Can you work these out from the model? Positions are in its coordinate system, mm. A direction names the side the tool comes from. Round coordinates to 2 decimals unless told otherwise and drop trailing zeros. Write each loop counter-clockwise with the first axis right and the second up, starting at its lowest first coordinate (ties: lowest second). Pieces come first, ordered by that corner, then holes. Notation, with made-up numbers: M 52,33 L 100,33 A20 ccw 100,72 Z; hole C -39.5,67 d5. An arc over 180 degrees is marked long. Answer in a Markdown table with one row per item. Add a question column.
(1) I'm going to push a flat-ended pin straight in: pin 1 (23 mm diameter, centred on x = 4, y = -7, fed in from +Z). Where does the tip first touch, or does it pass through?
(2) If I drill on probe 1 along Z at (x, y) = (-9, -10.5); probe 2 along Y at (x, z) = (14.5, -28.5); probe 3 along X at (y, z) = (0, -47), over which ranges is the centre line in solid material (lowest first)?
(3) Suppose I cut it at A-A, the plane z = -31. Write out the boundary of the cut face in (x, y).
(4) If we mould it in two halves opening along Y, with no side actions, what happens to faces 5 (the face through (-18, 24.25, -52)), 6 (the face through (-18, -24.25, -52)), 7 (the face through (-1, 0, -135)), 8 (the face through (-21.245, 0.467, -115.172))? For each: released by +Y, released by -Y, zero draft, split by the parting line, or undercut.
(5) Suppose I cut it at B-B, the plane x = 7. Count the separate pieces of the cut face and the enclosed holes in it, then the cut area to 3 significant figures.
(6) For faces 1 (the face through (22, 0, -32.5)), 2 (the face through (1, 0, -130)), 3 (the face through (-21.23, 0.93, -20.04)), 4 (the face through (-26.25, 0, -67)), which set-ups out of +Z, -Z, +X, -X, +Y, -Y let a thin tool reach every point of the face, with its end or its side?
(7) Suppose I cut it at C-C, the plane z = -80. Write out the boundary of the cut face in (x, y).
from build123d import *

# Parameters (mm, degrees)
F1_DEPTH      = 135
F2_R          = 21.25
F3_DEPTH      = 130
F4_W          = 24.25
F4_H          = 97.5
F5_DEPTH      = 50.1
F5_DEPTH_BACK = 25
F6_R          = 1.49999
F7_T3_DEPTH   = 141.00001
F7_T6_DEPTH   = 56
F7_T9_DEPTH   = 141.00001
F8_T1_DEPTH   = 28.5
F8_T4_ANGLE   = 180


# Not quite as in the source:
# - a fillet or chamfer that OpenCascade refuses, or shapes differently, is made with other operations: its cross-section is extruded or revolved along the edge and cut away or added
# - a fillet or chamfer is up to 0.001 mm smaller than in the source, because OpenCascade refuses the exact size


with BuildPart() as f1:
    # F0 (on Top) → F1 (new body)
    with BuildSketch(Plane.XY):
        with BuildLine():
            ThreePointArc((0, -24.25), (17.1473394438, -17.1473394438), (24.25, 0))
            ThreePointArc((24.25, 0), (17.1473394438, 17.1473394438), (0, 24.25))
            ThreePointArc((0, 24.25), (-24.25, 0), (0, -24.25))
        make_face()
        with BuildLine():
            ThreePointArc((0, -24.25), (-24.25, 0), (0, 24.25))
            Line((0, 24.25), (-26.25, 24.25))
            Line((-26.25, 24.25), (-26.25, -24.25))
            Line((-26.25, -24.25), (0, -24.25))
        make_face()
    extrude(amount=-F1_DEPTH)

    # F2 (on face) → F3 (cut)
    with BuildSketch(Plane.XY):
        Circle(F2_R)
    extrude(amount=-F3_DEPTH, mode=Mode.SUBTRACT)

    # F4 (on face) → F5 (cut, two sides)
    with BuildSketch(Plane.XZ.offset(24.25)) as f5_sk:
        with Locations((12.125, -81.25)):
            Rectangle(F4_W, F4_H)
        with BuildLine():
            Line((0, -130), (0, -32.5))
            ThreePointArc((0, -32.5), (-22.2460263089, -81.25), (0, -130))
        make_face()
    extrude(amount=-F5_DEPTH, mode=Mode.SUBTRACT)
    extrude(f5_sk.sketch, amount=F5_DEPTH_BACK, mode=Mode.SUBTRACT)

    # F6 (radius 1.5 in the source; OpenCascade refuses exactly that, so slightly less here)
    f6_edges = [f1.edges().sort_by_distance(p)[0] for p in [
        (24.25, 0, 0),
        (-13.125, -24.25, 0),
        (-13.125, 24.25, 0),
        (-26.25, 0, 0),
        (-21.25, 0, 0),
    ]]
    fillet(f6_edges, radius=F6_R)

    # F7: fillet of radius 1.5 on 4 edges, made by hand


with BuildPart() as f7_tool1:
    # F7_s2 → F7_t3 (new body)
    with BuildSketch(Plane.XY.offset(2.25001)):
        with BuildLine():
            ThreePointArc((-24.75, 24.25), (-25.8106601718, 23.8106601718), (-26.25, 22.75))
            Line((-26.25, 22.75), (-26.25, 24.25))
            Line((-26.25, 24.25), (-24.75, 24.25))
        make_face()
    extrude(amount=-F7_T3_DEPTH)


with BuildPart() as f7_tool4:
    # F7_s5 → F7_t6 (new body)
    with BuildSketch(Plane.XZ.offset(-28)):
        with BuildLine():
            ThreePointArc((-26.25, -133.5), (-25.8106601718, -134.5606601718), (-24.75, -135))
            Line((-24.75, -135), (-26.25, -135))
            Line((-26.25, -135), (-26.25, -133.5))
        make_face()
    extrude(amount=F7_T6_DEPTH)


with BuildPart() as f7_tool7:
    # F7_s8 → F7_t9 (new body)
    with BuildSketch(Plane.XY.offset(2.25001)):
        with BuildLine():
            ThreePointArc((-24.75, -24.25), (-25.8106601718, -23.8106601718), (-26.25, -22.75))
            Line((-26.25, -22.75), (-26.25, -24.25))
            Line((-26.25, -24.25), (-24.75, -24.25))
        make_face()
    extrude(amount=-F7_T9_DEPTH)


with BuildPart() as f1_1:
    add(f1.part)

    # F7_t10: cut F7_tool1, F7_tool4, F7_tool7
    add([f7_tool1.part, f7_tool4.part, f7_tool7.part], mode=Mode.SUBTRACT)

    # F8: fillet of radius 1.5 on 4 edges, made by hand

    # F8_s2 → F8_t1 (cut)
    with BuildSketch(Plane.YZ.offset(-28.5)):
        with BuildLine():
            ThreePointArc((-24.25, -133.5), (-23.8106601718, -134.5606601718), (-22.75, -135))
            Line((-22.75, -135), (-24.25, -135))
            Line((-24.25, -135), (-24.25, -133.5))
        make_face()
        with BuildLine():
            ThreePointArc((24.25, -133.5), (23.8106601718, -134.5606601718), (22.75, -135))
            Line((22.75, -135), (24.25, -135))
            Line((24.25, -135), (24.25, -133.5))
        make_face()
    extrude(amount=F8_T1_DEPTH, mode=Mode.SUBTRACT)

    # F8_s3 → F8_t4 (revolve, cut)
    with BuildSketch(Plane.YZ):
        with BuildLine():
            ThreePointArc((-24.25, -133.5), (-23.8106601718, -134.5606601718), (-22.75, -135))
            Line((-22.75, -135), (-24.25, -135))
            Line((-24.25, -135), (-24.25, -133.5))
        make_face()
    revolve(axis=Axis((0, 0, -135), (0, 0, 1)), revolution_arc=F8_T4_ANGLE, mode=Mode.SUBTRACT)


solid = f1_1.part
Calculated:
| question | item | result |
|---|---|---|
| 1 | pin 1 | z = -130 |
| 2 | probe 1 | -135 to -130 |
| 2 | probe 2 | -19.44 to -15.53, 15.53 to 19.44 |
| 2 | probe 3 | -26.25 to -21.25 |
| 3 | outline | M -26.25,-22.75 A1.5 ccw -24.75,-24.25 L 0,-24.25 A24.25 ccw 0,24.25 L -24.75,24.25 A1.5 ccw -26.25,22.75 Z; hole C 0,0 d42.5 |
| 4 | face 5 | released by +Y |
| 4 | face 6 | released by -Y |
| 4 | face 7 | zero draft |
| 4 | face 8 | undercut |
| 5 | separate pieces | 3 |
| 5 | enclosed holes | 0 |
| 5 | area | 434 mm² |
| 6 | face 1 | +X, +Y, -Y |
| 6 | face 2 | +X |
| 6 | face 3 | +Z |
| 6 | face 4 | +Z, -Z, -X, +Y, -Y |
| 7 | outline | M -26.25,-22.75 A1.5 ccw -24.75,-24.25 L -22.23,-24.25 L -22.23,24.25 L -24.75,24.25 A1.5 ccw -26.25,22.75 Z |
